Verification items for the finished model (mm, model axes). Face numbers are marked on the shaded views. A direction names the side the tool comes from. Give positions to 0.01 mm unless a question says otherwise; leave off trailing zeros. Write each loop counter-clockwise with the first axis right and the second up, starting at its lowest first coordinate (ties: lowest second). Pieces come first, ordered by that corner, then holes. Notation, with made-up numbers: (18, -7) -> (50, -7) arc R25 ccw to (50, 14) -> close; hole circle Ø10 at (64, 25.25). An arc over 180 degrees is marked (long way). Write item = value, one per line.
from build123d import *

# Parameters (mm, degrees)
SKETCH1_W           = 60
SKETCH1_H           = 28
SKETCH1_R           = 4.1
SKETCH1_R_2         = 1.6
BOSS_EXTRUDE1_DEPTH = 10
SKETCH2_R           = 11
CUT_EXTRUDE1_DEPTH  = 7.5


with BuildPart() as part:
    # Sketch1 → Boss-Extrude1 (new body)
    with BuildSketch(Plane.XY):
        Rectangle(SKETCH1_W, SKETCH1_H)
        with Locations((12.5, 0)):
            Circle(SKETCH1_R, mode=Mode.SUBTRACT)
        with Locations((-12.5, 0)):
            Circle(SKETCH1_R, mode=Mode.SUBTRACT)
        with Locations((-26.464466094, 10.464466094)):
            Circle(SKETCH1_R_2, mode=Mode.SUBTRACT)
        with Locations((-26.464466094, -10.464466094)):
            Circle(SKETCH1_R_2, mode=Mode.SUBTRACT)
        with Locations((26.464466094, -10.464466094)):
            Circle(SKETCH1_R_2, mode=Mode.SUBTRACT)
        with Locations((26.464466094, 10.464466094)):
            Circle(SKETCH1_R_2, mode=Mode.SUBTRACT)
    extrude(amount=BOSS_EXTRUDE1_DEPTH)

    # Sketch2 → Cut-Extrude1 (cut)
    with BuildSketch(Plane.XY.offset(10)):
        with Locations((-12.5, 0)):
            Circle(SKETCH2_R)
    extrude(amount=-CUT_EXTRUDE1_DEPTH, mode=Mode.SUBTRACT)


solid = part.part
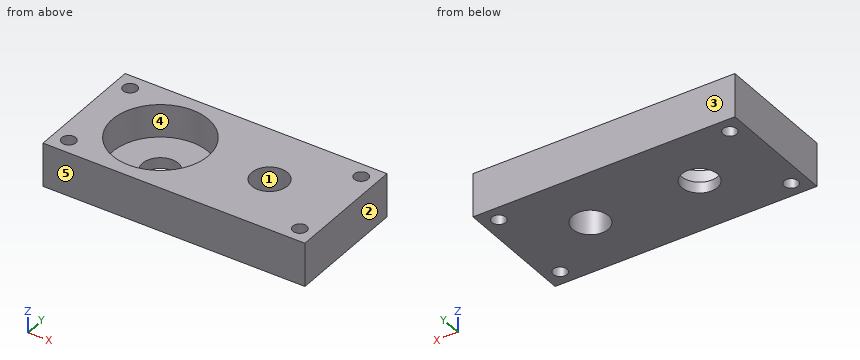
Item 1: Material ranges on line 1 (Y direction, x = -12.5, z = 0.95); line 2 (X direction, y = 2.25, z = 3.5); line 3 (Y direction, x = -12.5, z = 6.5), recorded low to high.
Response values:
line_1 = -14 to -4.1, 4.1 to 14
line_2 = -30 to -23.27, -1.73 to 9.07, 15.93 to 30
line_3 = -14 to -11, 11 to 14
Item 2: Sectioned sample at B-B on y = 0. Record the cut outline in (x, z).
Response values:
outline = (-30, 0) -> (-16.6, 0) -> (-16.6, 2.5) -> (-23.5, 2.5) -> (-23.5, 10) -> (-30, 10) -> close; (-8.4, 0) -> (8.4, 0) -> (8.4, 10) -> (-1.5, 10) -> (-1.5, 2.5) -> (-8.4, 2.5) -> close; (16.6, 0) -> (30, 0) -> (30, 10) -> (16.6, 10) -> close
Item 3: Set-up check for the marked faces 4 and 5: record each of +Z, -Z, +X, -X, +Y, -Y from which the full face is reachable in a straight line by a thin tool's end or side.
Response values:
face_4 = +Z
face_5 = +Z, -Z, +X, -X, -Y
Item 4: Sectioned sample at D-D on x = -12.5. Record the cut outline in (y, z).
Response values:
outline = (-14, 0) -> (-4.1, 0) -> (-4.1, 2.5) -> (-11, 2.5) -> (-11, 10) -> (-14, 10) -> close; (4.1, 0) -> (14, 0) -> (14, 10) -> (11, 10) -> (11, 2.5) -> (4.1, 2.5) -> close
Item 5: Mould release check, pull along Y, two halves, no side actions. Record for the marked faces 1, 2 and 3: +Y half, -Y half, draft (parallel to the pull), parting line (faces both ways), or undercut.
Response values:
face_1 = undercut
face_2 = draft
face_3 = +Y half
Item 6: Sectioned sample at C-C on z = 5. Record the cut outline in (x, y), then the cut area to 3 significant figures.
Response values:
outline = (-30, -14) -> (30, -14) -> (30, 14) -> (-30, 14) -> close; hole circle Ø3.2 at (-26.46, -10.46); hole circle Ø3.2 at (-26.46, 10.46); hole circle Ø22 at (-12.5, 0); hole circle Ø8.2 at (12.5, 0); hole circle Ø3.2 at (26.46, -10.46); hole circle Ø3.2 at (26.46, 10.46)
area = 1,210 mm^2
Item 7: Go/stop test with flat-tipped pins: P1, Ø10, axis at x = 5, y = -7, coming from the -Z side; P2, Ø13, axis at x = -12.5, y = 0, coming from the +Z side. Record where each tip stops, or that it passes through.
Response values:
P1 = 0
P2 = 2.5
Item 8: Sectioned sample at A-A on x = 12.5. Record the cut outline in (y, z).
Response values:
outline = (-14, 0) -> (-4.1, 0) -> (-4.1, 10) -> (-14, 10) -> close; (4.1, 0) -> (14, 0) -> (14, 10) -> (4.1, 10) -> close
